Can you work these out from the model? Positions are in its coordinate system, mm. A direction names the side the tool comes from. Coordinates: 2 decimals unless noted, no trailing zeros. Loops run counter-clockwise (first coordinate to the right, second up) from the corner with the lowest first, then second, coordinate; pieces in that order, holes last.
```python
from build123d import *

# Parameters (mm, degrees)
SKETCH5_R           = 16
BOSS_EXTRUDE1_DEPTH = 1
BOSS_EXTRUDE7_DEPTH = 1
BOSS_EXTRUDE8_DEPTH = 1
CIRPATTERN1_COUNT   = 2


with BuildPart() as part:
    # Sketch5 → Boss-Extrude1 (new body)
    with BuildSketch(Plane.XY):
        Circle(SKETCH5_R)
        with BuildLine():
            Line((-0.5, -14.991664351), (0.5, -14.991664351))
            ThreePointArc((0.5, -14.991664351), (10.606601718, -10.606601718), (14.991664351, -0.5))
            Line((14.991664351, -0.5), (14.991664351, 0.5))
            ThreePointArc((14.991664351, 0.5), (10.606601718, 10.606601718), (0.5, 14.991664351))
            Line((0.5, 14.991664351), (-0.5, 14.991664351))
            ThreePointArc((-0.5, 14.991664351), (-10.606601718, 10.606601718), (-14.991664351, 0.5))
            Line((-14.991664351, 0.5), (-14.991664351, -0.5))
            ThreePointArc((-14.991664351, -0.5), (-10.606601718, -10.606601718), (-0.5, -14.991664351))
        make_face(mode=Mode.SUBTRACT)
    extrude(amount=BOSS_EXTRUDE1_DEPTH)

    # Sketch6 → Boss-Extrude7 (add)
    with BuildSketch(Plane.XY):
        with BuildLine():
            Line((-11.661770518, 10.954593027), (-10.97567443, 10.224214923))
            ThreePointArc((-10.97567443, 10.224214923), (-10.628744174, 10.58441294), (-10.269999326, 10.932845642))
            Line((-10.269999326, 10.932845642), (-10.954665948, 11.661702018))
            ThreePointArc((-10.954665948, 11.661702018), (-11.313743872, 11.313673126), (-11.661770518, 10.954593027))
        make_face()
    boss_extrude7 = extrude(amount=-BOSS_EXTRUDE7_DEPTH)

    # Sketch8 → Boss-Extrude8 (add)
    with BuildSketch(Plane(origin=(0, 0, -1), x_dir=(-1, 0, 0), z_dir=(0, 0, -1))):
        Polygon((10.97567443, 10.224214923), (10.269999326, 10.932845642), (11.687165216, 12.344100701), (12.39284032, 11.635469982), align=None)
    boss_extrude8 = extrude(amount=BOSS_EXTRUDE8_DEPTH)

    # CirPattern1: Boss-Extrude7, Boss-Extrude8 ×2 about axis
    cirpattern1_axis = Axis((0, 0, 0), (0, 0, 1))
    for i in range(1, CIRPATTERN1_COUNT):
        add(boss_extrude7.rotate(cirpattern1_axis, i * 360 / CIRPATTERN1_COUNT))
        add(boss_extrude8.rotate(cirpattern1_axis, i * 360 / CIRPATTERN1_COUNT))


solid = part.part
```
Item 1: On a 3-axis mill with a long thin cutter (end or side, diameter ignored), from which of +Z, -Z, +X, -X, +Y, -Y can I reach the whole of each face in a straight line? I mean faces 1 (the face through (10.72, 10.49, 0.49)), 2 (the face through (11.694, -10.94, -1.493)), 3 (the face through (-11.694, 10.94, -1.493)). Say none if no direction works.
Results are:
face 1: +Z, -Z
face 2: -Z, +X, +Y
face 3: -Z, -X, -Y
Item 2: I'm going to push flat-ended pins straight in: P1, Ø1.5, axis at y = 8, z = -1, coming from the +X side; P2, Ø1.1, axis at x = -12, y = 11.5, coming from the +Z side; P3, Ø1, axis at x = 2.5, z = 0.5, coming from the -Y side; P4, Ø1.5, axis at y = -5, z = 0, coming from the +X side. Where does each tip first touch, or does it pass through?
Results are:
P1: passes through
P2: stops at z = -1
P3: stops at y = -15.87
P4: stops at x = 15.43
Item 3: I need wall thicknesses on line 1 along X through (y, z) = (0.5, 0.5); line 2 along X through (y, z) = (10, 0.6); line 3 along Y through (x, z) = (11, 0.1). Which ranges of each line are inside material? Lowest first, please.
Results are:
line 1: x = -15.99 to -14.99, 14.99 to 15.99
line 2: x = -12.49 to -11.18, 11.18 to 12.49
line 3: y = -11.62 to -10.2, 10.2 to 11.62
Item 4: We'd pull the mould along Y, two halves only. Please class faces 4 (the face through (10.97, -11.63, -1.49)), 5 (the face through (-11, 11, -2)), 6 (the face through (-14.992, 0, 0.5)): +Y half, -Y half, draft (parallel to the pull), parting line (faces both ways), or undercut.
Results are:
face 4: -Y half
face 5: draft
face 6: undercut
Item 5: Suppose I cut it at B-B, the plane y = 0. Please give me the cut outline in (x, z).
Results are:
outline: (-16, 0) - (-14.99, 0) - (-14.99, 1) - (-16, 1) - close; (14.99, 0) - (16, 0) - (16, 1) - (14.99, 1) - close
Item 6: Suppose I cut it at A-A, the plane z = -0.55. Please give me the cut outline in (x, y).
Results are:
outline: (-11.66, 10.95) - (-10.98, 10.22) arc R15 cw to (-10.27, 10.93) - (-10.95, 11.66) arc R16 ccw to start; (10.27, -10.93) - (10.95, -11.66) arc R16 ccw to (11.66, -10.95) - (10.98, -10.22) arc R15 cw to start
